For this review, take the finished solid that the model builds, in its own axes (mm). Face numbers are marked on the shaded views. Coordinates: 2 decimals unless noted, no trailing zeros. Order: outer loops, then holes, each group sorted by start corner. A loop starts at its lowest first (then second) coordinate and runs counter-clockwise, first axis right, second up. Notation, with made-up numbers: (67.25, 66.5) -> (86.25, 66.5) arc R32 ccw to (86.25, 103.5) -> close; hole circle Ø7 at (-34, 8.25). An arc over 180 degrees is marked (long way). Return JSON: item names as keys, results as strings. Group by question number.
Item 1: Take a section at C-C (x = 46.5). Write out the cut boundary in (y, z), then the cut area to 3 significant figures.
Item 2: Take a section at A-A (y = 31). Write out the cut boundary in (x, z).
Item 3: Draft analysis for pull direction Y (two halves, no side actions). For the marked faces 1, 2 and 3, state which applies: +Y half, -Y half, draft (parallel to the pull), parting line (faces both ways), or undercut.
Item 4: For line 1 along Y through (x, z) = (45, 37); line 2 along Y through (x, z) = (53, 32.5); line 3 along X through (y, z) = (22, 26.5), list the stretches that pass through material, from the lowest coordinate up.
Item 5: Insertion check: pin 1 (24 mm diameter, centred on x = 45, y = 31, fed in from -Z); pin 2 (5 mm diameter, centred on x = 61, y = 52, fed in from -Z); pin 3 (6 mm diameter, centred on y = 52, z = 26.5, fed in from +X); pin 4 (1.5 mm diameter, centred on y = 55.5, z = 22.5, fed in from +X). Each pin has a flat end and moves straight along its axis. Give the tip position at first contact, or say it passes through.
Item 6: Take a section at D-D (y = 11.5). Write out the cut boundary in (x, z), then the cut area to 3 significant figures.
Item 7: Take a section at B-B (z = 39). Write out the cut boundary in (x, y), then the cut area to 3 significant figures.
```python
from build123d import *

# Parameters (mm, degrees)
SKETCH1_R           = 15
BOSS_EXTRUDE2_DEPTH = 50
FILLET1_R           = 3.5
FILLET2_R           = 3.5
FILLET3_R           = 3.5


with BuildPart() as part:
    # Sketch1 → Boss-Extrude2 (new body)
    with BuildSketch(Plane.XY):
        Polygon((0, 0), (89.999999993, 0.001126334), (44.999024562, 77.942849502), align=None)
        with Locations((45, 31)):
            Circle(SKETCH1_R, mode=Mode.SUBTRACT)
    extrude(amount=BOSS_EXTRUDE2_DEPTH)

    # Fillet1
    fillet1_edges = [part.edges().sort_by_distance(p)[0] for p in [
        (44.999024562, 77.942849502, 25),
    ]]
    fillet(fillet1_edges, radius=FILLET1_R)

    # Fillet2
    fillet2_edges = [part.edges().sort_by_distance(p)[0] for p in [
        (89.999999993, 0.001126334, 25),
    ]]
    fillet(fillet2_edges, radius=FILLET2_R)

    # Fillet3
    fillet3_edges = [part.edges().sort_by_distance(p)[0] for p in [
        (0, 0, 25),
    ]]
    fillet(fillet3_edges, radius=FILLET3_R)


solid = part.part
```
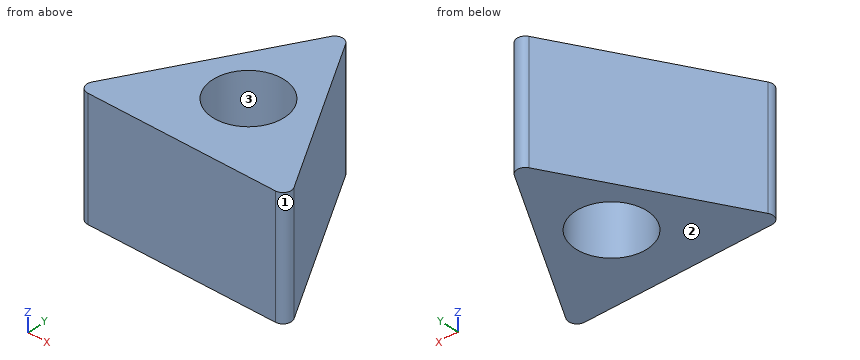
Findings below:
{
 "1": {"outline": "(0, 0) -> (16.08, 0) -> (16.08, 50) -> (0, 50) -> close; (45.92, 0) -> (74.1, 0) -> (74.1, 50) -> (45.92, 50) -> close", "area": "2,210 mm2"},
 "2": {"outline": "(17.9, 0) -> (30, 0) -> (30, 50) -> (17.9, 50) -> close; (60, 0) -> (72.1, 0) -> (72.1, 50) -> (60, 50) -> close"},
 "3": {"face 1": "parting line", "face 2": "draft", "face 3": "undercut"},
 "4": {"line 1": "y = 0 to 16, 46 to 74.44", "line 2": "y = 0 to 18.31, 43.69 to 64.09", "line 3": "x = 12.7 to 33, 57 to 77.3"},
 "5": {"pin 1": "passes through", "pin 2": "stops at z = 0", "pin 3": "stops at x = 61.71", "pin 4": "stops at x = 58.39"},
 "6": {"outline": "(6.64, 0) -> (83.36, 0) -> (83.36, 50) -> (6.64, 50) -> close", "area": "3,840 mm2"},
 "7": {"outline": "(3.03, 5.25) arc R3.5 ccw to (6.06, 0) -> (83.94, 0) arc R3.5 ccw to (86.97, 5.25) -> (48.03, 72.69) arc R3.5 ccw to (41.97, 72.69) -> close; hole circle Ø30 at (45, 31)", "area": "2,780 mm2"}
}
